Design review of the part built by this model. Coordinates are the model's own, in mm. A direction names the side the tool comes from. Round coordinates to 2 decimals unless told otherwise and drop trailing zeros. Loops run counter-clockwise (first coordinate to the right, second up) from the corner with the lowest first, then second, coordinate; pieces in that order, holes last. Notation, with made-up numbers: (83, 88.5) - (127, 88.5) arc R12 ccw to (127, 101.5) - close; hole circle Ø8 at (41, 88.25). An arc over 180 degrees is marked (long way). Return JSON: item names as keys, results as strings. Group by question number.
(1) We need section B-B, the plane x = 21. Write out the cut boundary in (y, z), and give its area (3 significant figures).
(2) For faces 5 (the flat face through (31, -22, 4)), 6 (the flat face through (-2, -43.4, -2)), 7 (the cylindrical face through (-0.59, -1.27, 4.46)), list the 3-axis set-ups (+Z, -Z, +X, -X, +Y, -Y) from which the entire face can be reached by the end or side of a thin tool; tool diameter is ignored.
(3) We need section D-D, the plane y = 9.5. Write out the cut boundary in (x, z).
(4) Clearance check with flat-ended pins moving along their axes: pin 1 (1.5 mm diameter, centred on x = 20, y = -9.5, fed in from -Z); pin 2 (3 mm diameter, centred on x = 3, y = 2, fed in from -Z); pin 3 (1.5 mm diameter, centred on x = 26, z = 4, fed in from +Y); pin 4 (8.5 mm diameter, centred on x = 21, y = -9.2, fed in from -Z). State where each tip first meets the part, or that it passes through.
(5) We need section A-A, the plane y = -34.2. Write out the cut boundary in (x, z), and give its area (3 significant figures).
(6) Wall thickness on L1, parallel to Y at x = 21, z = 2.15; L2, parallel to Y at x = 27, z = 3; L3, parallel to Z at x = 13.5, y = -14.5: over which ranges is each line inside the solid? List them lowest first. Write a range as [from, to].
(7) The part is to be moulded in two halves that separate along X. For faces 1 (the cylindrical face through (4.197, -0.419, 1.322)), 2 (the conical face through (17.75, -8.176, 2.408)), 3 (the flat face through (0, 36.8, 0)), 4 (the conical face through (21.44, -30.82, 2.41)), say which applies: pulls with the +X half, pulls with the -X half, needs draft (parallel to the pull), parting line crosses it, or undercut.
from build123d import *

# Parameters (mm, degrees)
EXTRUDE1_DEPTH       = 40
HOLEWZD1_D           = 6.5
HOLEWZD1_DEPTH       = 11
HOLEWZD1_CSINK_D     = 13
HOLEWZD1_CSINK_ANGLE = 90
CHAMFER1_SIZE        = 0.5


with BuildPart() as part:
    # Sketch1 → Extrude1 (new body)
    with BuildSketch(Plane.XZ.offset(41.7)):
        with BuildLine():
            Line((31, 5.5), (0, 5.5))
            ThreePointArc((0, 5.5), (-3.102418411, -4.541475531), (5.123475383, 2))
            Line((5.123475383, 2), (31, 2))
            Line((31, 2), (31, 5.5))
        make_face()
    extrude(amount=-EXTRUDE1_DEPTH)

    # Sketch2 → Revolve1 (revolve)
    with BuildSketch(Plane.XY):
        Polygon((2.5, 36.8), (0, 36.8), (0, -1.7), (4.5, -1.7), (4.5, -0.85), (4.4, -0.85), (4.4, 0), (2.5, 0), align=None)
    revolve(axis=Axis((0, 36.8, 0), (0, -1, 0)))

    # Sketch3 → Revolve2 (revolve)
    with BuildSketch(Plane.XY):
        Polygon((4.5, -41.7), (0, -41.7), (0, -44.9), (2.5, -44.9), (2.5, -43.4), (4.4, -43.4), (4.4, -42.55), (4.5, -42.55), align=None)
    revolve(axis=Axis((0, -41.7, 0), (0, -1, 0)))

    # HoleWzd1
    with Locations(Plane.XY.offset(5.5)):
        with Locations((21, -34.2), (21, -9.2)):
            CounterSinkHole(HOLEWZD1_D / 2, HOLEWZD1_CSINK_D / 2, depth=HOLEWZD1_DEPTH, counter_sink_angle=HOLEWZD1_CSINK_ANGLE)

    # Chamfer1
    chamfer1_edges = [part.edges().sort_by_distance(p)[0] for p in [
        (-2.5, 36.8, 0),
        (-2.5, -44.9, 0),
    ]]
    chamfer(chamfer1_edges, length=CHAMFER1_SIZE)


solid = part.part
Solutions:
{
 "1": {"outline": "(-41.7, 2) - (-37.45, 2) - (-37.45, 2.25) - (-40.7, 5.5) - (-41.7, 5.5) - close; (-30.95, 2) - (-12.45, 2) - (-12.45, 2.25) - (-15.7, 5.5) - (-27.7, 5.5) - (-30.95, 2.25) - close; (-5.95, 2) - (-1.7, 2) - (-1.7, 5.5) - (-2.7, 5.5) - (-5.95, 2.25) - close", "area": "73.4 mm^2"},
 "2": {"face 5": "+Z, -Z, +X, +Y, -Y", "face 6": "-Y", "face 7": "+Y"},
 "3": {"outline": "circle Ø5 at (0, 0)"},
 "4": {"pin 1": "through", "pin 2": "z = -2", "pin 3": "y = -1.7", "pin 4": "z = 2"},
 "5": {"outline": "(0, 5.5) arc R5.5 ccw (long way) to (5.12, 2) - (17.75, 2) - (17.75, 2.25) - (14.5, 5.5) - close; (24.25, 2) - (31, 2) - (31, 5.5) - (27.5, 5.5) - (24.25, 2.25) - close", "area": "157 mm^2"},
 "6": {"L1": "[-41.7, -37.45], [-30.95, -12.45], [-5.95, -1.7]", "L2": "[-41.7, -1.7]", "L3": "[2, 5.5]"},
 "7": {"face 1": "parting line crosses it", "face 2": "undercut", "face 3": "needs draft", "face 4": "undercut"}
}
